```python
from build123d import *

# Parameters (mm, degrees)
SKETCH1_W           = 109.8
SKETCH1_H           = 150
SKETCH1_R           = 42
SKETCH1_R_2         = 3.3
BOSS_EXTRUDE1_DEPTH = 12.7
CUT_EXTRUDE1_DEPTH  = 94.809914188
BOSS_EXTRUDE2_DEPTH = 12.7
FILLET1_R           = 12.8


with BuildPart() as part:
    # Sketch1 → Boss-Extrude1 (new body)
    with BuildSketch(Plane.XY):
        Rectangle(SKETCH1_W, SKETCH1_H)
        Circle(SKETCH1_R, mode=Mode.SUBTRACT)
        with Locations((-35.355339059, 35.355339059)):
            Circle(SKETCH1_R_2, mode=Mode.SUBTRACT)
        with Locations((35.355339059, 35.355339059)):
            Circle(SKETCH1_R_2, mode=Mode.SUBTRACT)
        with Locations((35.355339059, -35.355339059)):
            Circle(SKETCH1_R_2, mode=Mode.SUBTRACT)
        with Locations((-35.355339059, -35.355339059)):
            Circle(SKETCH1_R_2, mode=Mode.SUBTRACT)
    extrude(amount=BOSS_EXTRUDE1_DEPTH)

    # Sketch2 → Cut-Extrude1 (cut, through all)
    with BuildSketch(Plane(origin=(0, 0, 0), x_dir=(-1, 0, 0), z_dir=(0, 0, -1))):
        Polygon((-38.65, -75), (-32.05, -75), (-32.05, -70.3), (-29.686, -70.3), (-29.686, -64.46), (-32.05, -64.46), (-32.05, -59.76), (-38.65, -59.76), (-38.65, -64.46), (-41.014, -64.46), (-41.014, -70.3), (-38.65, -70.3), align=None)
        Polygon((32.05, -75), (32.05, -70.3), (29.686, -70.3), (29.686, -64.46), (32.05, -64.46), (32.05, -59.76), (38.65, -59.76), (38.65, -64.46), (41.014, -64.46), (41.014, -70.3), (38.65, -70.3), (38.65, -75), align=None)
    extrude(amount=-CUT_EXTRUDE1_DEPTH, mode=Mode.SUBTRACT)

    # Sketch4 → Boss-Extrude2 (add)
    with BuildSketch(Plane.XZ.offset(75)):
        Polygon((0, 0), (15.875, 0), (15.875, 12.7), (-15.875, 12.7), (-15.875, 0), align=None)
    extrude(amount=BOSS_EXTRUDE2_DEPTH)

    # Fillet1
    fillet1_edges = [part.edges().sort_by_distance(p)[0] for p in [
        (-54.9, 75, 6.35),
        (54.9, 75, 6.35),
    ]]
    fillet(fillet1_edges, radius=FILLET1_R)


solid = part.part
```
Check sheet for the modelled part. Datum: model origin and axes. Units: mm. A direction names the side the tool comes from. Coordinates: 2 decimals unless noted, no trailing zeros. Loops run counter-clockwise (first coordinate to the right, second up) from the corner with the lowest first, then second, coordinate; pieces in that order, holes last. Notation, with made-up numbers: M -29,88.5 L 27,88.5 A7 ccw 27,96.5 Z; hole C 32.25,5 d4. An arc over 180 degrees is marked long. Answer as a JSON object with one key per item and string values.
1. Scan lines: L1, parallel to X at y = -64, z = 11; L2, parallel to Y at x = 0, z = 6.5; L3, parallel to Y at x = -31, z = 1.75. Record each from-to range of solid material in increasing order. Write a range as from..to.
Outcome:
{"L1": "-54.9..-38.65, -32.05..32.05, 38.65..54.9", "L2": "-87.7..-42, 42..75", "L3": "-75..-70.3, -64.46..-28.34, 28.34..75"}
2. Sectioned sample at B-B on x = 0. Record the cut outline in (y, z).
Outcome:
{"outline": "M -87.7,0 L -42,0 L -42,12.7 L -87.7,12.7 Z; M 42,0 L 75,0 L 75,12.7 L 42,12.7 Z"}
3. Sectioned sample at C-C on y = 18. Record the cut outline in (x, z).
Outcome:
{"outline": "M -54.9,0 L -37.95,0 L -37.95,12.7 L -54.9,12.7 Z; M 37.95,0 L 54.9,0 L 54.9,12.7 L 37.95,12.7 Z"}
4. Depth check by flat-ended pin: P1, Ø4, axis at x = -22.5, z = 8, coming from the -Y side; P2, Ø6.5, axis at y = -79, z = 9, coming from the -X side (3 decimals); P3, Ø2, axis at x = -34.5, z = 7.5, coming from the -Y side. Enter the tip coordinate at first touch or a pass-through.
Outcome:
{"P1": "y = -75", "P2": "x = -15.875", "P3": "y = -59.76"}
5. Sectioned sample at A-A on y = -72. Record the cut outline in (x, z).
Outcome:
{"outline": "M -54.9,0 L -38.65,0 L -38.65,12.7 L -54.9,12.7 Z; M -32.05,0 L 32.05,0 L 32.05,12.7 L -32.05,12.7 Z; M 38.65,0 L 54.9,0 L 54.9,12.7 L 38.65,12.7 Z"}
6. Release check for a two-part mould opening along Y. For faces 1 (the flat face through (-24, -75, 6)), 2 (the cylindrical face through (-33.581, 38.138, 6.261)), 3 (the cylindrical face through (-51.2, 71.2, 6.4)) record: pulls with the +Y half, pulls with the -Y half, needs draft (parallel to the pull), parting line crosses it, or undercut.
Outcome:
{"face 1": "pulls with the -Y half", "face 2": "undercut", "face 3": "pulls with the +Y half"}
7. Sectioned sample at D-D on z = 6.5. Count the separate pieces of the cut face and the enclosed holes in it, and give its area (3 significant figures).
Outcome:
{"separate pieces": "1", "enclosed holes": "5", "area": "10,900 mm²"}
8. Access from +Z, -Z, +X, -X, +Y, -Y to the whole of each face (thin tool, end or side, straight path). Record for faces 4 (the flat face through (29.686, -67, 6)), 5 (the cylindrical face through (51.1, 71.3, 6.4)), 6 (the flat face through (-38.65, -62, 6)), 7 (the flat face through (-47, -75, 6)).
Outcome:
{"face 4": "+Z, -Z", "face 5": "+Z, -Z, +X, +Y", "face 6": "+Z, -Z, -Y", "face 7": "+Z, -Z, -X, -Y"}
